For this review, take the finished solid that the model builds, in its own axes (mm). A direction names the side the tool comes from. Coordinates: 2 decimals unless noted, no trailing zeros. Loops run counter-clockwise (first coordinate to the right, second up) from the corner with the lowest first, then second, coordinate; pieces in that order, holes last.
1. Take a section at D-D, the plane x = 22. State the section outline as (y, z) points.
2. Take a section at C-C, the plane x = 3. State the section outline as (y, z) points.
3. Clearance check with a flat-ended pin moving along its axis: P1, Ø2, axis at x = 6.5, z = 1.5, coming from the +Y side. State where the tip first meets the part, or that it passes through.
4. Take a section at B-B, the plane z = 0. State the section outline as (x, y) points, then the cut area to 3 significant figures.
5. To check wall thickness, follow probe 1 along X at (y, z) = (-1.75, -3.25); probe 2 along X at (y, z) = (0, 1); probe 3 along X at (y, z) = (-4, 2.75). State the ranges of each line that lie inside material, in increasing order.
6. Take a section at A-A, the plane y = 0. State the section outline as (x, z) points, then the cut area to 3 significant figures.
7. Machinability: for faces 4 (the face through (50.493, 2.173, 2.835)), 5 (the face through (57, 0, 0)), which of the approach directions +Z, -Z, +X, -X, +Y, -Y give a long, thin tool a straight path to every point of the face, cutting with its end or side? Answer none if there is none.
8. Mouldability with a two-part tool opening along X and no side actions: class faces 1 (the face through (28.2, 4.88, 1.08)), 2 (the face through (0, 0, 0)), 3 (the face through (50, -2.2, -3.3)) as pulls with the +X half, pulls with the -X half, needs draft (parallel to the pull), parting line crosses it, or undercut.
Autodesk Inventor part; units mm, degrees
ref_plane "YZ Plane" through (0, 0, 0) normal (1, 0, 0) x (0, 1, 0)
ref_plane "XZ Plane" through (0, 0, 0) normal (0, 1, 0) x (-1, 0, 0)
ref_plane "XY Plane" through (0, 0, 0) normal (0, 0, 1) x (1, 0, 0)
sketch "Esboço2" plane through (0, 0, 0) normal (1, 0, 0) x (0, 1, 0)
  circle A0 centre (0, 0) radius 5
  dimension "d0" = 10
extrude "Extrusão1" add sketch "Esboço2" along normal blind 6
sketch "Esboço3" plane through (6, 0, 0) normal (1, 0, 0) x (0, 0, -1)
  circle A0 centre (0, 0) radius 5
  circle A1 centre (0, 0) radius 3.5719
  dimension "d3" = 7.1437
extrude "Extrusão2" add sketch "Esboço3" along normal blind 1 contours A1
sketch "Esboço4" plane through (7, 0, 0) normal (1, 0, 0) x (0, 0, -1)
  circle A0 centre (0, 0) radius 3.5719
  circle A1 centre (0, 0) radius 5
  dimension "d6" = 10
extrude "Extrusão3" add sketch "Esboço4" along normal blind 43 contours A0 | A1
sketch "Esboço8" plane through (50, 0, 0) normal (1, 0, 0) x (0, 0, -1)
  circle A0 centre (0, 0) radius 5
  circle A1 centre (0, 0) radius 3.5719
  dimension "d34" = 7.1437
extrude "Extrusão6" add sketch "Esboço8" along normal blind 1 contours A1
sketch "Esboço9" plane through (51, 0, 0) normal (1, 0, 0) x (0, 0, -1)
  circle A0 centre (0, 0) radius 3.5719
  circle A1 centre (0, 0) radius 5
  dimension "d39" = 10
extrude "Extrusão7" add sketch "Esboço9" along normal blind 6 contours A0 | A1
chamfer "Chanfro2" distance 0.5 angle 45 2 edges at (57, 0, 5) (0, -5, 0)
sketch "Esboço10" plane through (0, 0, 0) normal (0, 0, 1) x (1, 0, 0)
  line L0 (0, -4.5) -> (0, 4.5)
  point P0 (0, 0)
  point P1 (3, 0)
  dimension "d43" = 3
hole "Furo3" at (3, 0, 0) direction (0, 0, -1) diameter 3 end through all
hole "Furo4" at (3, 0, 0) direction (0, 0, 1) diameter 3 end through all
properties part number "pino_a3" material "Aço carbono"
Results list:
1. outline: circle Ø10 at (0, 0)
2. outline: (-1.5, -4.77) - (-1.5, 4.77) arc R5 ccw to start; (1.5, -4.77) arc R5 ccw to (1.5, 4.77) - close
3. P1: stops at y = 4.96
4. outline: (0, -4.5) - (0.5, -5) - (6, -5) - (6, -3.57) - (7, -3.57) - (7, -5) - (50, -5) - (50, -3.57) - (51, -3.57) - (51, -5) - (56.5, -5) - (57, -4.5) - (57, 4.5) - (56.5, 5) - (51, 5) - (51, 3.57) - (50, 3.57) - (50, 5) - (7, 5) - (7, 3.57) - (6, 3.57) - (6, 5) - (0.5, 5) - (0, 4.5) - close; hole circle Ø3 at (3, 0)
4. area: 557 mm2
5. probe 1: x = 0 to 6, 7 to 50, 51 to 57
5. probe 2: x = 0 to 1.5, 4.5 to 57
5. probe 3: x = 0.35 to 6, 7 to 50, 51 to 56.65
6. outline: (0, -4.5) - (0.5, -5) - (1.5, -5) - (1.5, 5) - (0.5, 5) - (0, 4.5) - close; (4.5, -5) - (6, -5) - (6, -3.57) - (7, -3.57) - (7, -5) - (50, -5) - (50, -3.57) - (51, -3.57) - (51, -5) - (56.5, -5) - (57, -4.5) - (57, 4.5) - (56.5, 5) - (51, 5) - (51, 3.57) - (50, 3.57) - (50, 5) - (7, 5) - (7, 3.57) - (6, 3.57) - (6, 5) - (4.5, 5) - close
6. area: 534 mm2
7. face 4: none
7. face 5: +Z, -Z, +X, +Y, -Y
8. face 1: needs draft
8. face 2: pulls with the -X half
8. face 3: undercut
